Answer from the drawing. Dimensions are ordinates in mm from the lowest x, y and z of the part. A direction names the side the tool comes from. Coordinates: 2 decimals unless noted, no trailing zeros. Write each loop counter-clockwise with the first axis right and the second up, starting at its lowest first coordinate (ties: lowest second). Pieces come first, ordered by that corner, then holes.
(1) The part is cut by section C-C, the plane x = 3. Determine the outline of the cut face in (y, z).
(2) Given pin 1 (2.5 mm diameter, centred on y = 32, z = 9.5, fed in from -X); pin 2 (3 mm diameter, centred on x = 2.5, y = 14, fed in from +Z); pin 3 (1.4 mm diameter, centred on x = 3, y = 36.25, fed in from +Z); pin 4 (2 mm diameter, centred on y = 9, z = 3, fed in from +X), each flat-ended and moving along its own axis, determine where each tip first touches the part or whether it passes through.
(3) Which of the six approach directions +Z, -Z, +X, -X, +Y, -Y give full straight-line access (tool end or side, diameter ignored) to the marked faces 1, 2 and 3?
(4) Determine the mould class of the marked faces 4, 5, 6 and 7 for opening direction Y: pulls with the +Y half, pulls with the -Y half, needs draft (parallel to the pull), parting line crosses it, or undercut.
(5) Straight lines are drawn through the part: line 1 along Y through (x, z) = (3, 7.9); line 2 along Y through (x, z) = (1.25, 5); line 3 along Y through (x, z) = (0.75, 9). For each, find the intervals that lie inside material, in ascending order.
(6) The part is cut by section B-B, the plane z = 6. Determine the outline of the cut face in (x, y).
(7) The part is cut by section D-D, the plane y = 36.25. Determine the outline of the cut face in (x, z), and give its area (3 significant figures).
(8) The part is cut by section A-A, the plane y = 23.3. Determine the outline of the cut face in (x, z), and give its area (3 significant figures).
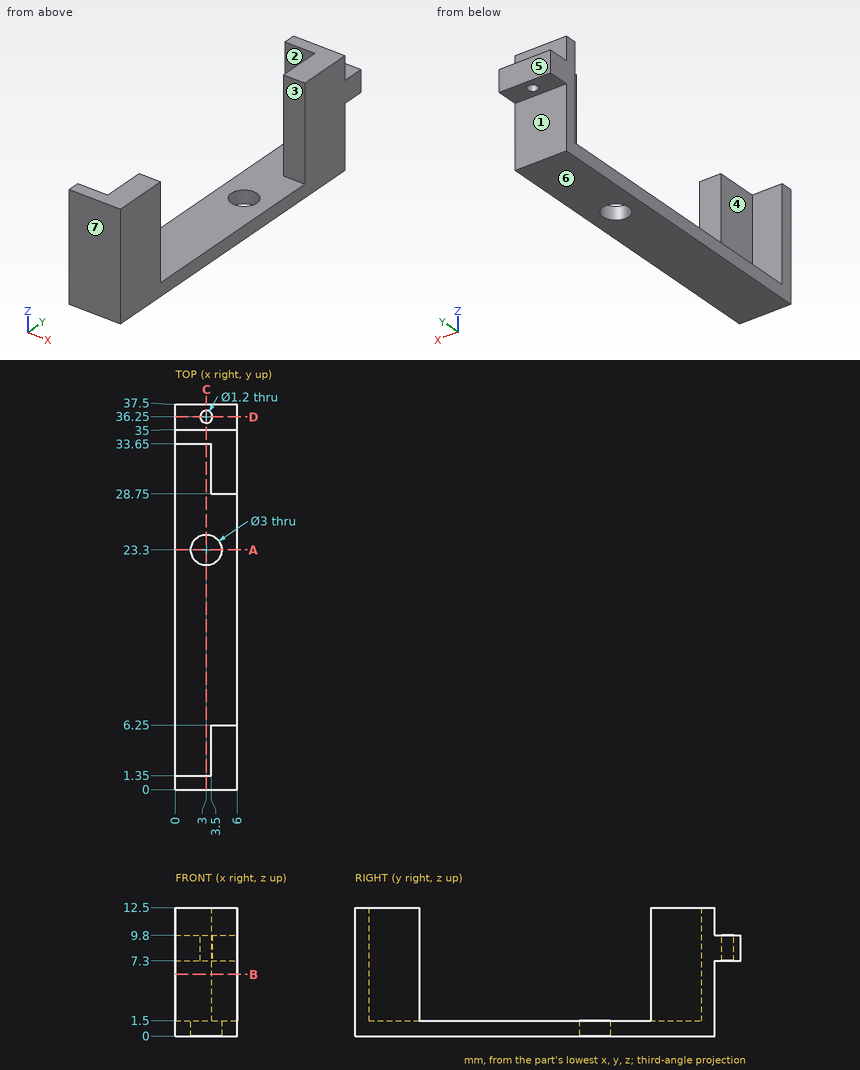
Computed:
1. outline: (0, 0) - (21.8, 0) - (21.8, 1.5) - (1.35, 1.5) - (1.35, 12.5) - (0, 12.5) - close; (24.8, 0) - (35, 0) - (35, 7.3) - (35.65, 7.3) - (35.65, 9.8) - (35, 9.8) - (35, 12.5) - (33.65, 12.5) - (33.65, 1.5) - (24.8, 1.5) - close; (36.85, 7.3) - (37.5, 7.3) - (37.5, 9.8) - (36.85, 9.8) - close
2. pin 1: stops at x = 3.5
2. pin 2: stops at z = 1.5
2. pin 3: stops at z = 9.8
2. pin 4: passes through
3. face 1: -Z, +X, -X, +Y
3. face 2: +Z, -X
3. face 3: +Z, +X, -X
4. face 4: undercut
4. face 5: pulls with the +Y half
4. face 6: needs draft
4. face 7: pulls with the -Y half
5. line 1: y = 0 to 1.35, 33.65 to 35.65, 36.85 to 37.5
5. line 2: y = 0 to 1.35, 33.65 to 35
5. line 3: y = 0 to 1.35, 33.65 to 37.5
6. outline: (0, 0) - (6, 0) - (6, 6.25) - (3.5, 6.25) - (3.5, 1.35) - (0, 1.35) - close; (0, 33.65) - (3.5, 33.65) - (3.5, 28.75) - (6, 28.75) - (6, 35) - (0, 35) - close
7. outline: (0, 7.3) - (2.4, 7.3) - (2.4, 9.8) - (0, 9.8) - close; (3.6, 7.3) - (6, 7.3) - (6, 9.8) - (3.6, 9.8) - close
7. area: 12.0 mm2
8. outline: (0, 0) - (1.5, 0) - (1.5, 1.5) - (0, 1.5) - close; (4.5, 0) - (6, 0) - (6, 1.5) - (4.5, 1.5) - close
8. area: 4.50 mm2
